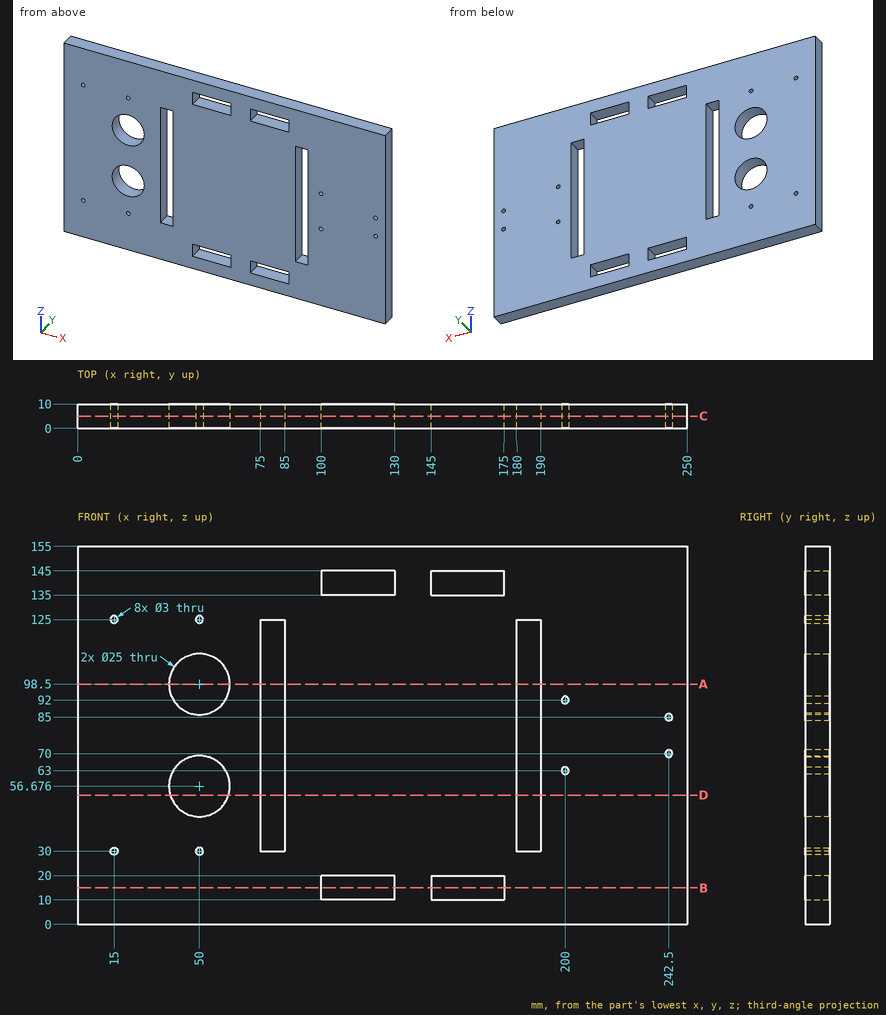
Verification items for this drawing (mm, ordinates from the low corner). Round coordinates to 2 decimals unless told otherwise and drop trailing zeros. Order: outer loops, then holes, each group sorted by start corner. A loop starts at its lowest first (then second) coordinate and runs counter-clockwise, first axis right, second up. Notation, with made-up numbers: M 20.5,-19.75 L 77.5,-19.75 A6 cw 77.5,-8.75 Z; hole C 65,-37 d3. An arc over 180 degrees is marked long. Answer in a Markdown table with one row per item. Add a question column.
Item 1: Sectioned sample at C-C, the plane y = 5. State how many separate pieces and enclosed holes the cut face has, plus the area to 3 significant figures.
Item 2: Sectioned sample at D-D, the plane z = 53. Enter the section's corners in (x, y), plus the area to 3 significant figures.
Item 3: Material ranges on L1, parallel to Z at x = 155.5, y = 2.5; L2, parallel to X at y = 6, z = 70; L3, parallel to Z at x = 200, y = 7.25, recorded low to high. Write a range as [from, to].
Item 4: Sectioned sample at B-B, the plane z = 15. Enter the section's corners in (x, y).
Item 5: Sectioned sample at A-A, the plane z = 98.5. Enter the section's corners in (x, y), plus the area to 3 significant figures.
Filled in:
| question | item | result |
|---|---|---|
| 1 | separate pieces | 1 |
| 1 | enclosed holes | 16 |
| 1 | area | 34,600 mm² |
| 2 | outline | M 0,0 L 38.05,0 L 38.05,10 L 0,10 Z; M 61.95,0 L 75,0 L 75,10 L 61.95,10 Z; M 85,0 L 180,0 L 180,10 L 85,10 Z; M 190,0 L 250,0 L 250,10 L 190,10 Z |
| 2 | area | 2,060 mm² |
| 3 | L1 | z = [0, 10], [20, 135], [145, 155] |
| 3 | L2 | x = [0, 75], [85, 180], [190, 241], [244, 250] |
| 3 | L3 | z = [0, 61.5], [64.5, 90.5], [93.5, 155] |
| 4 | outline | M 0,0 L 100,0 L 100,10 L 0,10 Z; M 130,0 L 145,0 L 145,10 L 130,10 Z; M 175,0 L 250,0 L 250,10 L 175,10 Z |
| 5 | outline | M 0,0 L 37.5,0 L 37.5,10 L 0,10 Z; M 62.5,0 L 75,0 L 75,10 L 62.5,10 Z; M 85,0 L 180,0 L 180,10 L 85,10 Z; M 190,0 L 250,0 L 250,10 L 190,10 Z |
| 5 | area | 2,050 mm² |
